```python
from build123d import *

# Parameters (mm, degrees)
SKETCH_1_R          = 8
SKETCH_1_R_2        = 2.6
EXTRUDE_215_DEPTH   = 2
EXTRUDE_8_120_DEPTH = 2


with BuildPart() as part:
    # 草图1 → Extrude 215 (new body)
    with BuildSketch(Plane.XY):
        Circle(SKETCH_1_R)
        Circle(SKETCH_1_R_2, mode=Mode.SUBTRACT)
    extrude(amount=EXTRUDE_215_DEPTH)

    # 草图2 → 8寸三叶桨轮廓_120度均布 (add)
    with BuildSketch(Plane.XY):
        Polygon((5, -4), (28, -10), (72, -9), (100, -2), (101.6, 0), (100, 2), (70, 5), (24, 8), (5, 4), align=None)
        Polygon((0.964101615, 6.330127019), (-5.339745962, 29.248711306), (-28.205771366, 66.853829072), (-48.267949192, 87.602540378), (-50.8, 87.988181024), (-51.732050808, 85.602540378), (-39.330127019, 58.121778265), (-18.92820323, 16.784609691), (-5.964101615, 2.330127019), align=None)
        Polygon((-5.964101615, -2.330127019), (-22.660254038, -19.248711306), (-43.794228634, -57.853829072), (-51.732050808, -85.602540378), (-50.8, -87.988181024), (-48.267949192, -87.602540378), (-30.669872981, -63.121778265), (-5.07179677, -24.784609691), (0.964101615, -6.330127019), align=None)
    extrude(amount=EXTRUDE_8_120_DEPTH)


solid = part.part
```
Work out the finished part from the listing and answer in its coordinate system (mm). A direction names the side the tool comes from. Round coordinates to 2 decimals unless told otherwise and drop trailing zeros. Write each loop counter-clockwise with the first axis right and the second up, starting at its lowest first coordinate (ties: lowest second). Pieces come first, ordered by that corner, then holes.
1) A cutting plane is placed at D-D on y = -34.5. Determine the outline of the cut face in (x, z), and give its area (3 significant figures).
2) A cutting plane is placed at B-B on x = -10.5. Determine the outline of the cut face in (y, z).
3) Which of the six approach directions +Z, -Z, +X, -X, +Y, -Y give full straight-line access (tool end or side, diameter ignored) to faces 5 (the face through (15.475, 6.205, 0.986)), 6 (the face through (-29.27, 37.74, 0.99)), 7 (the face through (3.917, -6.976, 0.986)), 8 (the face through (-4, 0, 0)), 9 (the face through (-18.05, -44.22, 0.99))?
4) A cutting plane is placed at C-C on x = 86. Determine the outline of the cut face in (y, z), and give its area (3 significant figures).
5) Flat-ended cylindrical pins translate along their axes: P1, Ø2, axis at x = -5, y = -18, coming from the -Z side; P2, Ø1, axis at x = -11, z = 0.5, coming from the -Y side; P3, Ø12, axis at x = 40, y = -20.5, coming from the -Z side. Find the tip coordinate at first contact, or state that the pin passes through.
6) A cutting plane is placed at A-A on z = 0.6. Determine the outline of the cut face in (x, y).
7) Determine the mould class of faces 1 (the face through (-47.708, -71.534, 0.986)), 2 (the face through (-45.618, 72.055, 0.986)), 3 (the face through (-4, 0, 2)), 4 (the face through (4.08, 6.88, 0.99)) for opening direction Y: pulls with the +Y half, pulls with the -Y half, needs draft (parallel to the pull), parting line crosses it, or undercut.
8) Consider probe 1 along Y at (x, z) = (-42, 0.7); probe 2 along Y at (x, z) = (1, 1.65); probe 3 along Y at (x, z) = (93.5, 1) (3 decimals). Determine where each line is inside the solid, lowest interval first.
Entries:
1. outline: (-31.01, 0) - (-11.56, 0) - (-11.56, 2) - (-31.01, 2) - close
1. area: 38.9 mm2
2. outline: (-32.91, 0) - (-6.93, 0) - (-6.93, 2) - (-32.91, 2) - close; (7.39, 0) - (37.74, 0) - (37.74, 2) - (7.39, 2) - close
3. face 5: +Z, -Z, +Y
3. face 6: +Z, -Z, -X
3. face 7: +Z, -Z, -Y
3. face 8: -Z, +X, -X, +Y, -Y
3. face 9: +Z, -Z, +X, -Y
4. outline: (-5.5, 0) - (3.4, 0) - (3.4, 2) - (-5.5, 2) - close
4. area: 17.8 mm2
5. P1: stops at z = 0
5. P2: stops at y = -34.41
5. P3: passes through
6. outline: (-51.73, -85.6) - (-50.8, -87.99) - (-48.27, -87.6) - (-30.67, -63.12) - (-5.07, -24.78) - (0.42, -7.99) arc R8 ccw to (6.66, -4.43) - (28, -10) - (72, -9) - (100, -2) - (101.6, 0) - (100, 2) - (70, 5) - (24, 8) - (6.71, 4.36) arc R8 ccw to (0.51, 7.98) - (-5.34, 29.25) - (-28.21, 66.85) - (-48.27, 87.6) - (-50.8, 87.99) - (-51.73, 85.6) - (-39.33, 58.12) - (-18.93, 16.78) - (-7.13, 3.63) arc R8 ccw to (-7.17, -3.55) - (-22.66, -19.25) - (-43.79, -57.85) - close; hole circle Ø5.2 at (0, 0)
7. face 1: undercut
7. face 2: undercut
7. face 3: needs draft
7. face 4: pulls with the +Y half
8. probe 1: y = -78.88 to -54.58, 64.04 to 81.12
8. probe 2: y = -7.94 to -2.4, 2.4 to 7.94
8. probe 3: y = -3.625 to 2.65
